Here's how the part is built. I have some questions about the finished solid (model axes, mm). A direction names the side the tool comes from. Give positions to 0.01 mm unless a question says otherwise; leave off trailing zeros. Order: outer loops, then holes, each group sorted by start corner. A loop starts at its lowest first (then second) coordinate and runs counter-clockwise, first axis right, second up. Notation, with made-up numbers: (55, 70.25) - (94, 70.25) arc R15 cw to (94, 98.25) - close; hole circle Ø11 at (-6, -34). An arc over 180 degrees is marked (long way). One line per question, with ' | ' between items.
from build123d import *

# Parameters (mm, degrees)
SKETCH_1_R          = 25
EXTRUDE_1_DEPTH     = 10
CUT_EXTRUDE_START   = 10
SKETCH_1_4_R        = 40
CUT_EXTRUDE_1_DEPTH = 1


with BuildPart() as part:
    # 草圖1 → 填料-伸長1 (new body)
    with BuildSketch(Plane.XY):
        with BuildLine():
            Line((-50, 0), (-50, -42))
            Line((-50, -42), (-40, -52))
            Line((-40, -52), (-20, -52))
            Line((-20, -52), (-20, -70))
            Line((-20, -70), (20, -70))
            Line((20, -70), (20, -52))
            Line((20, -52), (40, -52))
            Line((40, -52), (50, -42))
            Line((50, -42), (50, 0))
            ThreePointArc((50, 0), (0, 50), (-50, 0))
        make_face()
        Circle(SKETCH_1_R, mode=Mode.SUBTRACT)
    extrude(amount=EXTRUDE_1_DEPTH)

    # 草圖1<4> → 除料-伸長1 (cut)
    with BuildSketch(Plane.XY.offset(CUT_EXTRUDE_START)):
        Circle(SKETCH_1_4_R)
    extrude(amount=-CUT_EXTRUDE_1_DEPTH, mode=Mode.SUBTRACT)


solid = part.part
1) On a 3-axis mill with a long thin cutter (end or side, diameter ignored), from which of +Z, -Z, +X, -X, +Y, -Y can I reach the whole of each face in a straight line? I mean faces 4 (the face through (17.22, 18.34, 9)), 5 (the face through (20, -61, 5)), 6 (the face through (-30, -52, 5)). Say none if no direction works.
Model answer:
face 4: +Z | face 5: +Z, -Z, +X, -Y | face 6: +Z, -Z, -X, -Y
2) I want a section at A-A (x = -17). List the corners of the cut face in (y, z) for me, plus the area to 3 significant figures.
Model answer:
outline: (-70, 0) - (-18.33, 0) - (-18.33, 9) - (-36.21, 9) - (-36.21, 10) - (-70, 10) - close; (18.33, 0) - (47.02, 0) - (47.02, 10) - (36.21, 10) - (36.21, 9) - (18.33, 9) - close | area: 768 mm2
3) I want a section at B-B (y = 7). List the corners of the cut face in (x, z) for me.
Model answer:
outline: (-49.51, 0) - (-24, 0) - (-24, 9) - (-39.38, 9) - (-39.38, 10) - (-49.51, 10) - close; (24, 0) - (49.51, 0) - (49.51, 10) - (39.38, 10) - (39.38, 9) - (24, 9) - close
4) I want a section at C-C (z = 1.75). List the corners of the cut face in (x, y) for me.
Model answer:
outline: (-50, -42) - (-40, -52) - (-20, -52) - (-20, -70) - (20, -70) - (20, -52) - (40, -52) - (50, -42) - (50, 0) arc R50 ccw to (-50, 0) - close; hole circle Ø50 at (0, 0)
5) I'm going to push flat-ended pins straight in: P1, Ø1, axis at x = -37.5, z = 1.5, coming from the -Y side; P2, Ø5, axis at y = -64, z = 6, coming from the +X side; P3, Ø4, axis at x = -24.5, z = 9, coming from the +Y side. Where does each tip first touch, or does it pass through?
Model answer:
P1: stops at y = -52 | P2: stops at x = 20 | P3: stops at y = 44.65
6) Thinking about a two-plate mould opening in X: for faces 1 (the face through (-8.67, -39.05, 9.51)), 2 (the face through (50, -21, 5)), 3 (the face through (-50, -21, 5)), which applies, +X half, -X half, draft (parallel to the pull), parting line (faces both ways), or undercut?
Model answer:
face 1: undercut | face 2: +X half | face 3: -X half
7) Please list where these lines run through material, in increasing order: L1, parallel to X at y = -55.5, z = 2.5; L2, parallel to Y at x = 15.5, z = 8; L3, parallel to Z at x = -14.5, y = -32.5.
Model answer:
L1: x = -20 to 20 | L2: y = -70 to -19.62, 19.62 to 47.54 | L3: z = 0 to 9
8) I want a section at D-D (y = 34). List the corners of the cut face in (x, z) for me.
Model answer:
outline: (-36.66, 0) - (36.66, 0) - (36.66, 10) - (21.07, 10) - (21.07, 9) - (-21.07, 9) - (-21.07, 10) - (-36.66, 10) - close
